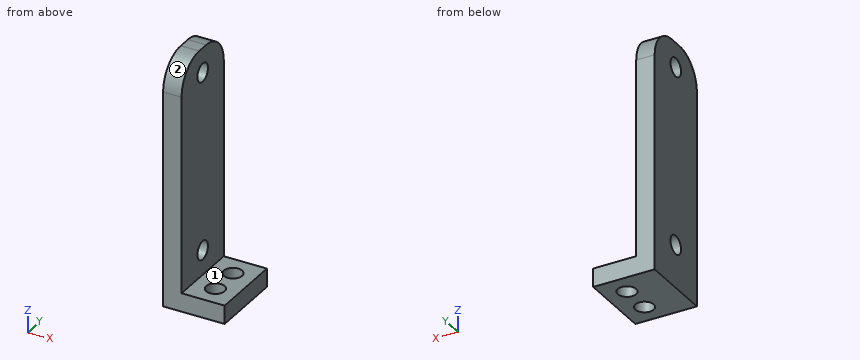
from build123d import *

# Parameters (mm, degrees)
CYLINDER003_R           = 1.5
CYLINDER003_DEPTH       = 10
CYLINDER003_PITCH_ANGLE = 90
CYLINDER002_R           = 1.5
CYLINDER002_DEPTH       = 10
CYLINDER002_PITCH_ANGLE = 90
BOX001_W                = 3
BOX001_H                = 12
BOX001_DEPTH            = 40
FILLET_R                = 5
CYLINDER001_R           = 1.5
CYLINDER001_DEPTH       = 10
CYLINDER_R              = 1.5
CYLINDER_DEPTH          = 10
BOX_W                   = 10
BOX_H                   = 12
BOX_DEPTH               = 3


with BuildPart() as cylinder003:
    # Cylinder003 → Cylinder003 (new body)
    with BuildSketch(Plane.XY):
        Circle(CYLINDER003_R)
    extrude(amount=CYLINDER003_DEPTH)


with BuildPart() as cylinder003_1:
    # Cylinder003 pitch: moved
    add(cylinder003.part.rotate(Axis((0, 0, 0), (0, 1, 0)), CYLINDER003_PITCH_ANGLE))


with BuildPart() as cylinder003_2:
    # Cylinder003 placement: moved
    add(cylinder003_1.part.moved(Location((0, 6, 36))))


with BuildPart() as cylinder002:
    # Cylinder002 → Cylinder002 (new body)
    with BuildSketch(Plane.XY):
        Circle(CYLINDER002_R)
    extrude(amount=CYLINDER002_DEPTH)


with BuildPart() as cylinder002_1:
    # Cylinder002 pitch: moved
    add(cylinder002.part.rotate(Axis((0, 0, 0), (0, 1, 0)), CYLINDER002_PITCH_ANGLE))


with BuildPart() as cylinder002_2:
    # Cylinder002 placement: moved
    add(cylinder002_1.part.moved(Location((0, 6, 7))))


with BuildPart() as cut003:
    # Box001 → Box001 (new body)
    with BuildSketch(Plane.XY):
        with Locations((1.5, 6)):
            Rectangle(BOX001_W, BOX001_H)
    extrude(amount=BOX001_DEPTH)

    # Fillet
    fillet_edges = [cut003.edges().sort_by_distance(p)[0] for p in [
        (1.5, 0, 40),
        (1.5, 12, 40),
    ]]
    fillet(fillet_edges, radius=FILLET_R)

    # Cut002: cut Cylinder002
    add(cylinder002_2.part, mode=Mode.SUBTRACT)

    # Cut003: cut Cylinder003
    add(cylinder003_2.part, mode=Mode.SUBTRACT)


with BuildPart() as cylinder001:
    # Cylinder001 → Cylinder001 (new body)
    with BuildSketch(Plane(origin=(6.5, 8.5, 0), x_dir=(1, 0, 0), z_dir=(0, 0, 1))):
        Circle(CYLINDER001_R)
    extrude(amount=CYLINDER001_DEPTH)


with BuildPart() as cylinder:
    # Cylinder → Cylinder (new body)
    with BuildSketch(Plane(origin=(6.5, 3.5, 0), x_dir=(1, 0, 0), z_dir=(0, 0, 1))):
        Circle(CYLINDER_R)
    extrude(amount=CYLINDER_DEPTH)


with BuildPart() as fusion:
    # Box → Box (new body)
    with BuildSketch(Plane.XY):
        with Locations((5, 6)):
            Rectangle(BOX_W, BOX_H)
    extrude(amount=BOX_DEPTH)

    # Cut: cut Cylinder
    add(cylinder.part, mode=Mode.SUBTRACT)

    # Cut001: cut Cylinder001
    add(cylinder001.part, mode=Mode.SUBTRACT)

    # Fusion: union Cut003
    add(cut003.part)


solid = fusion.part
Input: part model. Units: mm. Frame: model coordinates. Face numbers are marked on the shaded views. A direction names the side the tool comes from. Coordinates: 2 decimals unless noted, no trailing zeros. Loops run counter-clockwise (first coordinate to the right, second up) from the corner with the lowest first, then second, coordinate; pieces in that order, holes last.
Q1. Cut plane A-A (x = 6.5). Output: boundary loops of the cut face in (y, z).
Q2. Material intervals for line 1 (Y direction, x = 6.5, z = 1.5); line 2 (X direction, y = 8.5, z = 2); line 3 (Z direction, x = 1.5, y = 6.75), sorted ascending.
Q3. Set-up query: the marked faces 1 and 2. Return all of +Z, -Z, +X, -X, +Y, -Y with unobstructed straight access to the full face (end or side cutting, diameter ignored); none if empty.
Q4. Contact query for flat-ended pins moving along their axis: pin 1 (2.5 mm diameter, centred on x = 6.5, y = 3.5, fed in from -Z); pin 2 (3.5 mm diameter, centred on y = 6, z = 27, fed in from +X); pin 3 (1.5 mm diameter, centred on x = 2.5, y = 1.5, fed in from +Z). Output: stop coordinate, or through.
Q5. Cut plane C-C (y = 6). Output: boundary loops of the cut face in (x, z), then the cut area to 3 significant figures.
Q6. Cut plane B-B (z = 7). Output: boundary loops of the cut face in (x, y), then the cut area to 3 significant figures.
Q7. Cut plane D-D (x = 2). Output: boundary loops of the cut face in (y, z).
Working result:
1. outline: (0, 0) - (2, 0) - (2, 3) - (0, 3) - close; (5, 0) - (7, 0) - (7, 3) - (5, 3) - close; (10, 0) - (12, 0) - (12, 3) - (10, 3) - close
2. line 1: y = 0 to 2, 5 to 7, 10 to 12
2. line 2: x = 0 to 5, 8 to 10
2. line 3: z = 0 to 5.7, 8.3 to 34.7, 37.3 to 40
3. face 1: +Z, +X, +Y, -Y
3. face 2: +Z, +X, -X, -Y
4. pin 1: passes through
4. pin 2: stops at x = 3
4. pin 3: stops at z = 39.18
5. outline: (0, 0) - (10, 0) - (10, 3) - (3, 3) - (3, 5.5) - (0, 5.5) - close; (0, 8.5) - (3, 8.5) - (3, 34.5) - (0, 34.5) - close; (0, 37.5) - (3, 37.5) - (3, 40) - (0, 40) - close
5. area: 123 mm2
6. outline: (0, 0) - (3, 0) - (3, 4.5) - (0, 4.5) - close; (0, 7.5) - (3, 7.5) - (3, 12) - (0, 12) - close
6. area: 27.0 mm2
7. outline: (0, 0) - (12, 0) - (12, 35) arc R5 ccw to (7, 40) - (5, 40) arc R5 ccw to (0, 35) - close; hole circle Ø3 at (6, 7); hole circle Ø3 at (6, 36)
